```python
from build123d import *

# Parameters (mm, degrees)
SKETCH1_W           = 24.892
SKETCH1_H           = 7.874
BOSS_EXTRUDE1_DEPTH = 2.286
SKETCH8_R           = 1.8
CUT_EXTRUDE4_DEPTH  = 8.29
BOSS_EXTRUDE2_START = -8.29
SKETCH10_R          = 4
SKETCH10_R_2        = 1.925
BOSS_EXTRUDE2_DEPTH = 8.2
CHAMFER1_START      = -15.87596875
CHAMFER1_DEPTH      = 8.2
SKETCH11_W          = 8.402
SKETCH11_H          = 2.286
SKETCH11_W_2        = 8.29
CUT_EXTRUDE5_DEPTH  = 1


with BuildPart() as part:
    # Sketch1 → Boss-Extrude1 (new body)
    with BuildSketch(Plane.XY):
        with Locations((-11.83196875, 3.65678125)):
            Rectangle(SKETCH1_W, SKETCH1_H)
    extrude(amount=BOSS_EXTRUDE1_DEPTH)

    # Sketch8 → Cut-Extrude4 (cut)
    with BuildSketch(Plane(origin=(0, 0, 0), x_dir=(-1, 0, 0), z_dir=(0, 0, -1))):
        with Locations((6.78496875, 3.09378125)):
            Circle(SKETCH8_R)
        with Locations((16.78496875, 3.09378125)):
            Circle(SKETCH8_R)
    extrude(amount=-CUT_EXTRUDE4_DEPTH, mode=Mode.SUBTRACT)

    # Sketch10 → Boss-Extrude2 (add)
    with BuildSketch(Plane(origin=(0.61403125, 0, 0), x_dir=(0, 0, -1), z_dir=(1, 0, 0)).offset(BOSS_EXTRUDE2_START)):
        with Locations((-1.143, 11.426998045)):
            Circle(SKETCH10_R)
        with Locations(Location((-1.143, 11.426998045, 0), (0, 0, 90))):
            Circle(SKETCH10_R_2, mode=Mode.SUBTRACT)
    extrude(amount=-BOSS_EXTRUDE2_DEPTH)

    # Chamfer1: read off the stored shape, not the designer's step
    # Chamfer1 outline → Chamfer1 (add)
    with BuildSketch(Plane.YZ.offset(CHAMFER1_START)):
        with BuildLine():
            Line((8.88905951, 4.234741902), (5.314022428, 2.286))
            Line((5.314022428, 2.286), (7.59378125, 2.286))
            ThreePointArc((7.59378125, 2.286), (8.095736451, 3.357203285), (8.88905951, 4.234741902))
        make_face()
    extrude(amount=CHAMFER1_DEPTH)

    # Sketch11 → Cut-Extrude5 (cut)
    with BuildSketch(Plane(origin=(0, 7.59378125, 0), x_dir=(1, 0, 0), z_dir=(0, 1, 0))):
        with Locations((-20.07696875, -1.143)):
            Rectangle(SKETCH11_W, SKETCH11_H)
        with Locations((-3.53096875, -1.143)):
            Rectangle(SKETCH11_W_2, SKETCH11_H)
    extrude(amount=-CUT_EXTRUDE5_DEPTH, mode=Mode.SUBTRACT)


solid = part.part
```
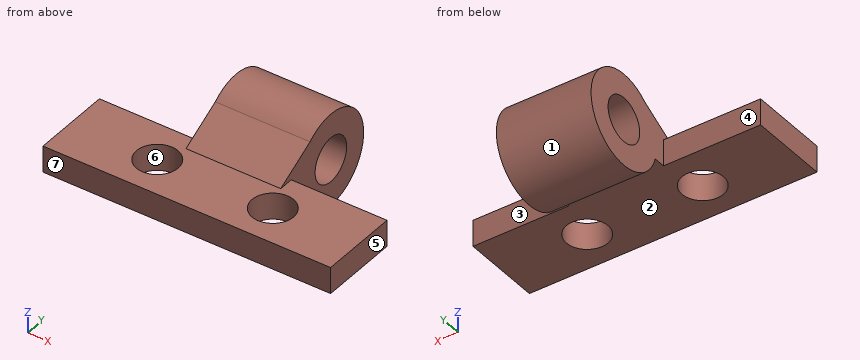
Verification items for the finished model (mm, model axes). Face numbers are marked on the shaded views. A direction names the side the tool comes from. Round coordinates to 2 decimals unless told otherwise and drop trailing zeros. Write each loop counter-clockwise with the first axis right and the second up, starting at its lowest first coordinate (ties: lowest second). Pieces come first, ordered by that corner, then holes. Notation, with made-up numbers: (72.25, -26.75) -> (95.25, -26.75) arc R28 cw to (95.25, -3.75) -> close; hole circle Ø6 at (63, 15.5). An arc over 180 degrees is marked (long way). Write each question's results on one line, items separated by ' | '. Start each with the question number.
1. Cross-section at B-B (y = 12.5). Enter the section's corners in (x, z).
2. Material ranges on probe 1 along Y at (x, z) = (-12.25, 1.25); probe 2 along X at (y, z) = (9.75, 4.25); probe 3 along Z at (x, y) = (-6.25, 6.25), recorded low to high. Write a range as from..to.
3. Cross-section at D-D (x = -13). Enter the section's corners in (y, z) (3 decimals), then the cut area to 3 significant figures.
4. Set-up check for the marked faces 1, 2, 3 and 4: record each of +Z, -Z, +X, -X, +Y, -Y from which the full face is reachable in a straight line by a thin tool's end or side.
5. Cross-section at A-A (z = 2.75). Enter the section's corners in (x, y), then the cut area to 3 significant figures.
6. Cross-section at C-C (y = 4). Enter the section's corners in (x, z), then the cut area to 3 significant figures.
7. Depth check by flat-ended pin: P1, Ø3, axis at x = -7.5, z = 4, coming from the +Y side; P2, Ø8.5, axis at x = -12, y = 2, coming from the -Z side; P3, Ø2.5, axis at y = 9.5, z = 0, coming from the -X side; P4, Ø3, axis at x = -16.78, y = 3.09, coming from the +Z side. Enter the tip coordinate at first touch or a pass-through.
8. Draft check along X on the marked faces 5, 6 and 7. Enter one of: +X half, -X half, draft (parallel to the pull), parting line (faces both ways), or undercut.
Solutions:
1) outline: (-15.88, -2.71) -> (-7.68, -2.71) -> (-7.68, -0.46) -> (-15.88, -0.46) -> close; (-15.88, 2.74) -> (-7.68, 2.74) -> (-7.68, 5) -> (-15.88, 5) -> close
2) probe 1: y = -0.28..9.5, 13.35..15.43 | probe 2: x = -15.88..-7.68 | probe 3: z = 0..2.29
3) outline: (-0.28, 0) -> (7.594, 0) arc R4 ccw (long way) to (8.889, 4.235) -> (5.314, 2.286) -> (-0.28, 2.286) -> close; hole circle Ø3.85 at (11.427, 1.143) | area: 58.3 mm2
4) face 1: +X, -X | face 2: -Z, +X, -X, -Y | face 3: +Z, -Z, +X, +Y | face 4: +Z, -Z, -X, +Y
5) outline: (-15.88, 6.17) -> (-7.68, 6.17) -> (-7.68, 10.37) -> (-15.88, 10.37) -> close; (-15.88, 12.49) -> (-7.68, 12.49) -> (-7.68, 15.09) -> (-15.88, 15.09) -> close | area: 55.8 mm2
6) outline: (-24.28, 0) -> (-18.34, 0) -> (-18.34, 2.29) -> (-24.28, 2.29) -> close; (-15.23, 0) -> (-8.34, 0) -> (-8.34, 2.29) -> (-15.23, 2.29) -> close; (-5.23, 0) -> (0.61, 0) -> (0.61, 2.29) -> (-5.23, 2.29) -> close | area: 42.7 mm2
7) P1: stops at y = 15.19 | P2: stops at z = 0 | P3: stops at x = -15.88 | P4: passes through
8) face 5: +X half | face 6: undercut | face 7: draft
